```python
from build123d import *

# Parameters (mm, degrees)
SKETCH_1_W          = 49.5
SKETCH_1_H          = 21
EXTRUDE_1_DEPTH     = 30.4
SKETCH_2_W          = 19
SKETCH_2_H          = 2.5
EXTRUDE_2_DEPTH     = 7
SKETCH_3_W          = 49.5
SKETCH_3_H          = 21
EXTRUDE_3_DEPTH     = 7
SKETCH_4_R          = 3
CUT_EXTRUDE_1_DEPTH = 7
SKETCH_5_R          = 4
EXTRUDE_4_DEPTH     = 5.4
FILLET_1_R          = 1
FILLET_2_R          = 1
FILLET_3_R          = 1
FILLET_4_R          = 1
FILLET_5_R          = 1
FILLET_6_R          = 1
FILLET_7_R          = 1
FILLET_8_R          = 1


with BuildPart() as part:
    # 草图1 → 凸台-拉伸1 (new body)
    with BuildSketch(Plane(origin=(0, 0, 0), x_dir=(1, 0, 0), z_dir=(0, 1, 0))):
        Rectangle(SKETCH_1_W, SKETCH_1_H)
    extrude(amount=EXTRUDE_1_DEPTH)

    # 草图2 → 凸台-拉伸2 (add)
    with BuildSketch(Plane(origin=(24.75, 0, 0), x_dir=(0, 0, -1), z_dir=(1, 0, 0))):
        with Locations((0, 29.15)):
            Rectangle(SKETCH_2_W, SKETCH_2_H)
    extrude_2 = extrude(amount=EXTRUDE_2_DEPTH)

    # 草图3 → 凸台-拉伸3 (add)
    with BuildSketch(Plane(origin=(0, 30.4, 0), x_dir=(1, 0, 0), z_dir=(0, 1, 0))):
        Rectangle(SKETCH_3_W, SKETCH_3_H)
    extrude(amount=EXTRUDE_3_DEPTH)

    # 草图4 → 切除-拉伸1 (cut)
    with BuildSketch(Plane(origin=(0, 30.4, 0), x_dir=(1, 0, 0), z_dir=(0, 1, 0))):
        with Locations((29.25, 5)):
            Circle(SKETCH_4_R)
        with Locations((29.25, -5)):
            Circle(SKETCH_4_R)
    cut_extrude_1 = extrude(amount=-CUT_EXTRUDE_1_DEPTH, mode=Mode.SUBTRACT)

    # 草图5 → 凸台-拉伸4 (add)
    with BuildSketch(Plane(origin=(0, 37.4, 0), x_dir=(1, 0, 0), z_dir=(0, 1, 0))):
        with Locations(Location((14.45, 0, 0), (0, 0, 90))):
            Circle(SKETCH_5_R)
    extrude(amount=EXTRUDE_4_DEPTH)

    # 镜向2: 凸台-拉伸2, 切除-拉伸1 across plane
    add(extrude_2.mirror(Plane(origin=(0, 0, 0), x_dir=(0, 0, 1), z_dir=(1, 0, 0))))
    add(cut_extrude_1.mirror(Plane(origin=(0, 0, 0), x_dir=(0, 0, 1), z_dir=(1, 0, 0))), mode=Mode.SUBTRACT)

    # 圆角1
    fillet_1_edges = [part.edges().sort_by_distance(p)[0] for p in [
        (24.75, 18.7, -10.5),
    ]]
    fillet(fillet_1_edges, radius=FILLET_1_R - 0.0001)  # a hair under: the kernel refuses the full size

    # 圆角2
    fillet_2_edges = [part.edges().sort_by_distance(p)[0] for p in [
        (24.75, 18.7, 10.5),
    ]]
    fillet(fillet_2_edges, radius=FILLET_2_R - 0.0001)  # a hair under: the kernel refuses the full size

    # 圆角3
    fillet_3_edges = [part.edges().sort_by_distance(p)[0] for p in [
        (-24.75, 18.7, 10.5),
    ]]
    fillet(fillet_3_edges, radius=FILLET_3_R - 0.0001)  # a hair under: the kernel refuses the full size

    # 圆角4
    fillet_4_edges = [part.edges().sort_by_distance(p)[0] for p in [
        (-24.75, 18.7, -10.5),
    ]]
    fillet(fillet_4_edges, radius=FILLET_4_R - 0.0001)  # a hair under: the kernel refuses the full size

    # 圆角5
    fillet_5_edges = [part.edges().sort_by_distance(p)[0] for p in [
        (-31.75, 29.15, -9.5),
    ]]
    fillet(fillet_5_edges, radius=FILLET_5_R)

    # 圆角6
    fillet_6_edges = [part.edges().sort_by_distance(p)[0] for p in [
        (-31.75, 29.15, 9.5),
    ]]
    fillet(fillet_6_edges, radius=FILLET_6_R)

    # 圆角7
    fillet_7_edges = [part.edges().sort_by_distance(p)[0] for p in [
        (31.75, 29.15, 9.5),
    ]]
    fillet(fillet_7_edges, radius=FILLET_7_R)

    # 圆角8
    fillet_8_edges = [part.edges().sort_by_distance(p)[0] for p in [
        (31.75, 29.15, -9.5),
    ]]
    fillet(fillet_8_edges, radius=FILLET_8_R)


solid = part.part
```
The listing builds one solid part. Answer for the finished solid, in the listing's coordinates (mm). A direction names the side the tool comes from. Give positions to 0.01 mm unless a question says otherwise; leave off trailing zeros. Write each loop counter-clockwise with the first axis right and the second up, starting at its lowest first coordinate (ties: lowest second). Pieces come first, ordered by that corner, then holes. Notation, with made-up numbers: M 81,52.5 L 130,52.5 A27 ccw 130,75.5 Z; hole C 25.25,81.25 d11. An arc over 180 degrees is marked long. Write each question's results on one line, items separated by ' | '.
Q1. Flat-ended cylindrical pins translate along their axes: P1, Ø10.5, axis at x = 9.5, z = -0.5, coming from the +Y side; P2, Ø4, axis at x = -3, z = 7, coming from the +Y side; P3, Ø7, axis at x = -29.25, z = -5, coming from the -Y side; P4, Ø4, axis at y = 32.5, z = 7.5, coming from the -X side. Find the tip coordinate at first contact, or state that the pin passes through.
Output values:
P1: y = 42.8 | P2: y = 37.4 | P3: y = 27.9 | P4: x = -24.75
Q2. Section B-B, the plane z = 5 is taken. Write down the section's boundary in (x, y).
Output values:
outline: M -26.25,27.9 L -24.75,27.9 L -24.75,0 L 24.75,0 L 24.75,27.9 L 26.25,27.9 L 26.25,30.4 L 24.75,30.4 L 24.75,37.4 L -24.75,37.4 L -24.75,30.4 L -26.25,30.4 Z
Q3. Section D-D, the plane y = 16.5 is taken. Write down the section's boundary in (x, z).
Output values:
outline: M -24.75,-9.5 A1 ccw -23.75,-10.5 L 23.75,-10.5 A1 ccw 24.75,-9.5 L 24.75,9.5 A1 ccw 23.75,10.5 L -23.75,10.5 A1 ccw -24.75,9.5 Z
Q4. For a pull along Z with two mould halves and no side action, classify faces 6 (the cylindrical face through (26.252, 29.167, 4.893)), 7 (the flat face through (27, 27.9, 0)), 8 (the flat face through (28, 29, -9.5)) as released by +Z, released by -Z, zero draft, split by the parting line, or undercut.
Output values:
face 6: undercut | face 7: zero draft | face 8: released by -Z
Q5. Section A-A, the plane x = 29.25 is taken. Write down the section's boundary in (y, z), then the cut area to 3 significant figures.
Output values:
outline: M 27.9,-9.5 L 30.4,-9.5 L 30.4,-8 L 27.9,-8 Z; M 27.9,-2 L 30.4,-2 L 30.4,2 L 27.9,2 Z; M 27.9,8 L 30.4,8 L 30.4,9.5 L 27.9,9.5 Z | area: 17.5 mm2
Q6. Consider L1, parallel to Z at x = -29, y = 29; L2, parallel to X at y = 8, z = -7.25; L3, parallel to Y at x = 21.5, z = 4.25. Determine where each line is inside the solid, lowest interval first. Write a range as from..to.
Output values:
L1: -9.5..-7.99, -2.01..2.01, 7.99..9.5 | L2: -24.75..24.75 | L3: 0..37.4
Q7. A tool of negligible diameter and unlimited length cuts with its end or side. For faces 1 (the flat face through (-27, 27.9, 0)), 2 (the flat face through (-28, 29, -9.5)), 3 (the flat face through (27, 30.4, 0)), 4 (the cylindrical face through (10.484, 40.062, 0.521)), 5 (the flat face through (31.75, 29, -8)), from which of +Z, -Z, +X, -X, +Y, -Y can it reach the whole face along a straight path? Write none if from no direction.
Output values:
face 1: +Z, -Z, -X, -Y | face 2: -Z, -X, +Y, -Y | face 3: +Z, -Z, +X, +Y | face 4: +Y | face 5: +Z, -Z, +X, +Y, -Y
Q8. Section C-C, the plane x = 14.45 is taken. Write down the section's boundary in (y, z), then the cut area to 3 significant figures.
Output values:
outline: M 0,-10.5 L 37.4,-10.5 L 37.4,-4 L 42.8,-4 L 42.8,4 L 37.4,4 L 37.4,10.5 L 0,10.5 Z | area: 829 mm2
